```python
from build123d import *

# Parameters (mm, degrees)
F0_W     = 100
F0_H     = 100
F1_DEPTH = 30
F2_R     = 10
F3_DEPTH = 100
F4_R     = 10
F5_DEPTH = 100
F6_W     = 98
F6_H     = 98
F7_DEPTH = 28
F8_R     = 10
F9_DEPTH = 3


# Not quite as in the source:
# - a feature names something its author has since deleted; it is built from what else it names


with BuildPart() as f1:
    # F0 (on Front) → F1 (new body)
    with BuildSketch(Plane.XZ):
        with Locations((25.5921050906, -0.9599315155)):
            Rectangle(F0_W, F0_H)
    extrude(amount=-F1_DEPTH)

    # F2 (on face) → F3 (cut)
    with BuildSketch(Plane.YZ.offset(75.5921050906)):
        with Locations((15, 24.0400684845)):
            Circle(F2_R)
        with Locations((15, -25.9599315155)):
            Circle(F2_R)
    extrude(amount=-F3_DEPTH, mode=Mode.SUBTRACT)

    # F4 (on face) → F5 (cut)
    with BuildSketch(Plane.XY.offset(49.0400684845)):
        with Locations((0, 15)):
            Circle(F4_R)
        with Locations((50.5921050906, 14.5671376958)):
            Circle(F4_R)
    extrude(amount=-F5_DEPTH, mode=Mode.SUBTRACT)

    # F6 (on face) → F7 (cut)
    with BuildSketch(Plane.XZ):
        with Locations((25.5921050906, -1.0704044253)):
            Rectangle(F6_W, F6_H)
    extrude(amount=-F7_DEPTH, mode=Mode.SUBTRACT)

    # F8 (on face) → F9 (cut)
    with BuildSketch(Plane(origin=(0, 30, 0), x_dir=(-1, 0, 0), z_dir=(0, 1, 0))):
        with Locations((0, -20.037606527)):
            Circle(F8_R)
        with Locations((0, 21.7908981225)):
            Circle(F8_R)
        with Locations((-25.5921050906, 0)):
            Circle(F8_R)
        with Locations((-50.5921050906, 24.0400684845)):
            Circle(F8_R)
        with Locations((-50.5921050906, -25.9599315155)):
            Circle(F8_R)
    extrude(amount=-F9_DEPTH, mode=Mode.SUBTRACT)


solid = f1.part
```
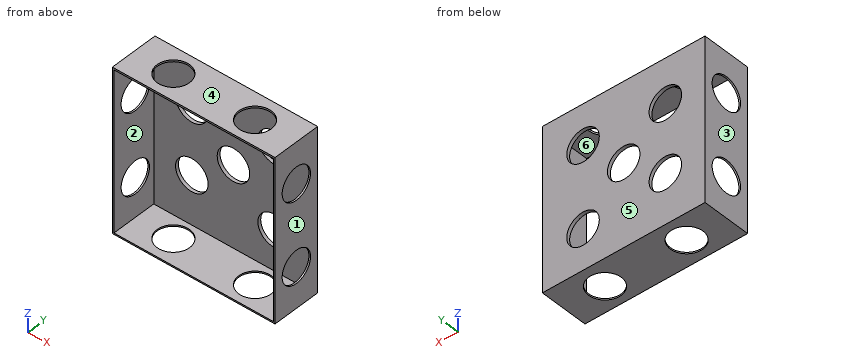
Can you work these out from the model? Positions are in its coordinate system, mm. Face numbers are marked on the shaded views. A direction names the side the tool comes from. Give positions to 0.01 mm unless a question says otherwise; leave off trailing zeros. Loops run counter-clockwise (first coordinate to the right, second up) from the corner with the lowest first, then second, coordinate; pieces in that order, holes last. Notation, with made-up numbers: M 66,58.25 L 118,58.25 A27 ccw 118,91.25 Z; hole C 8.5,-33.75 d8. An arc over 180 degrees is marked long. One line per question, with ' | ' between items. Start each with the question number.
Q1. If we section it at C-C (x = 68.5): Please give me the cut outline in (y, z).
Q2. If we mould it in two halves opening along X, with no side actions, what happens to the marked faces 1, 2, 3 and 4? For each: +X half, -X half, draft (parallel to the pull), parting line (faces both ways), or undercut.
Q3. If we section it at A-A (x = 0): Please give me the cut outline in (y, z), plus the area to 3 significant figures.
Q4. If I drill on line 1 (Z direction, x = -23.65, y = 15); line 2 (Z direction, x = 38, y = 9.25); line 3 (X direction, y = 6.75, z = -39), over which ranges is the centre line in solid material (lowest first)? Write a range as from..to.
Q5. If we section it at B-B (z = 0): Please give me the cut outline in (x, y), plus the area to 3 significant figures.
Q6. If we section it at D-D (z = 19): Please give me the cut outline in (x, y), plus the area to 3 significant figures.
Q7. For the marked faces 5 and 6, which set-ups out of +Z, -Z, +X, -X, +Y, -Y let a thin tool reach every point of the face, with its end or its side?
Computed:
1) outline: M 0,-50.96 L 30,-50.96 L 30,49.04 L 0,49.04 L 0,47.93 L 28,47.93 L 28,-50.07 L 0,-50.07 Z
2) face 1: +X half | face 2: undercut | face 3: -X half | face 4: draft
3) outline: M 0,-50.96 L 5,-50.96 L 5,-50.07 L 0,-50.07 Z; M 0,47.93 L 5,47.93 L 5,49.04 L 0,49.04 Z; M 25,-50.96 L 30,-50.96 L 30,-30.04 L 28,-30.04 L 28,-50.07 L 25,-50.07 Z; M 25,47.93 L 28,47.93 L 28,31.79 L 30,31.79 L 30,49.04 L 25,49.04 Z; M 28,-10.04 L 30,-10.04 L 30,11.79 L 28,11.79 Z | area: 136 mm²
4) line 1: z = -50.96..-35.96, -15.96..14.04, 34.04..49.04 | line 2: z = -50.96..-50.07, 47.93..49.04 | line 3: x = -24.41..-23.41, 74.59..75.59
5) outline: M -24.41,0 L -23.41,0 L -23.41,28 L 15.59,28 L 15.59,30 L -24.41,30 Z; M 35.59,28 L 74.59,28 L 74.59,0 L 75.59,0 L 75.59,30 L 35.59,30 Z | area: 216 mm²
6) outline: M -24.41,0 L -23.41,0 L -23.41,6.36 L -24.41,6.36 Z; M -24.41,23.64 L -23.41,23.64 L -23.41,28 L -9.6,28 L -9.6,30 L -24.41,30 Z; M 9.6,28 L 41.96,28 L 41.96,30 L 9.6,30 Z; M 59.23,28 L 74.59,28 L 74.59,23.64 L 75.59,23.64 L 75.59,30 L 59.23,30 Z; M 74.59,0 L 75.59,0 L 75.59,6.36 L 74.59,6.36 Z | area: 148 mm²
7) face 5: +Z, -Z, +X, -X, +Y | face 6: -Y
